Part model, mm, in its own coordinate system. Face numbers are marked on the shaded views. Round coordinates to 2 decimals unless told otherwise and drop trailing zeros. Loops run counter-clockwise (first coordinate to the right, second up) from the corner with the lowest first, then second, coordinate; pieces in that order, holes last. Notation, with made-up numbers: (11.25, 24.5) -> (60.25, 24.5) arc R27 ccw to (60.25, 63.5) -> close; hole circle Ø4 at (-32.75, 25.25). An arc over 180 degrees is marked (long way). Use a Markdown table: item, result. Add a question column.
Item 1: Probe line 1 (Z direction, x = 345, y = 43); line 2 (Y direction, x = 1050, z = -488.25); line 3 (Y direction, x = 960, z = -260). List the from-to ranges inside material, lowest first. Write a range as [from, to].
Item 2: Two-plate mould, pull along Z, no slides. Class the marked faces 1 and 2: pulls with the +Z half, pulls with the -Z half, needs draft (parallel to the pull), parting line crosses it, or undercut.
Item 3: Cut at A-A, the plane y = 30. List the corners of the cut face in (x, z).
Item 4: Cut at C-C, the plane x = 387.5. List the corners of the cut face in (y, z).
Item 5: Cut at B-B, the plane x = 1050. List the corners of the cut face in (y, z), plus the area to 3 significant figures.
Item 6: Flat gauge pin, fed straight in: pin 1 (1.5 mm diameter, centred on x = 274, z = -302.5, fed in from -Y). Where does the tip first touch, or does it go through?
Item 7: Cut at D-D, the plane z = -382. List the corners of the cut face in (x, y), plus the area to 3 significant figures.
```python
from build123d import *

# Parameters (mm, degrees)
SKETCH1_W           = 1200
SKETCH1_H           = 500
BOSS_EXTRUDE1_DEPTH = 68
SKETCH3_R           = 15
CUT_EXTRUDE2_DEPTH  = 1302.77724669
SKETCH4_R           = 15
CUT_EXTRUDE3_DEPTH  = 1302.77724669
SKETCH2_W           = 1200
SKETCH2_H           = 450
CUT_EXTRUDE1_DEPTH  = 50


with BuildPart() as part:
    # Sketch1 → Boss-Extrude1 (new body)
    with BuildSketch(Plane(origin=(0, 0, 0), x_dir=(1, 0, 0), z_dir=(0, 1, 0))):
        with Locations((600, 250)):
            Rectangle(SKETCH1_W, SKETCH1_H)
    extrude(amount=BOSS_EXTRUDE1_DEPTH)

    # Sketch3 → Cut-Extrude2 (cut, through all)
    with BuildSketch(Plane.XY):
        with Locations((150, 30)):
            Circle(SKETCH3_R)
    extrude(amount=-CUT_EXTRUDE2_DEPTH, mode=Mode.SUBTRACT)

    # Sketch4 → Cut-Extrude3 (cut, through all)
    with BuildSketch(Plane(origin=(0, 0, -500), x_dir=(-1, 0, 0), z_dir=(0, 0, -1))):
        with Locations((-1050, 30)):
            Circle(SKETCH4_R)
    extrude(amount=-CUT_EXTRUDE3_DEPTH, mode=Mode.SUBTRACT)

    # Sketch2 → Cut-Extrude1 (cut)
    with BuildSketch(Plane.XZ):
        with Locations((600, -250)):
            Rectangle(SKETCH2_W, SKETCH2_H)
    extrude(amount=-CUT_EXTRUDE1_DEPTH, mode=Mode.SUBTRACT)


solid = part.part
```
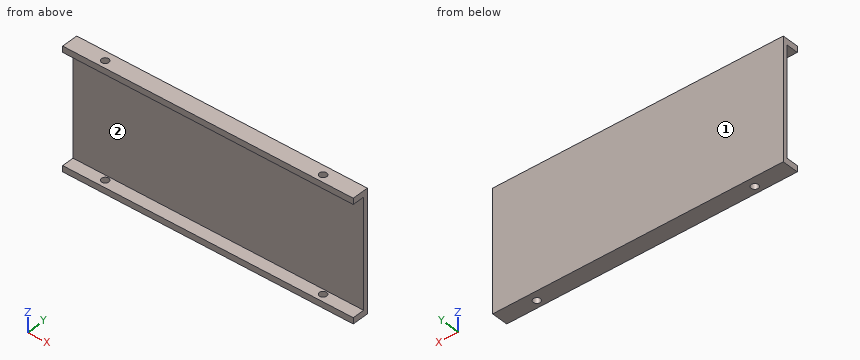
A:
| question | item | result |
|---|---|---|
| 1 | line 1 | z = [-500, -475], [-25, 0] |
| 1 | line 2 | y = [0, 15], [45, 68] |
| 1 | line 3 | y = [50, 68] |
| 2 | face 1 | needs draft |
| 2 | face 2 | undercut |
| 3 | outline | (0, -500) -> (135, -500) -> (135, -475) -> (0, -475) -> close; (0, -25) -> (135, -25) -> (135, 0) -> (0, 0) -> close; (165, -500) -> (1035, -500) -> (1035, -475) -> (165, -475) -> close; (165, -25) -> (1035, -25) -> (1035, 0) -> (165, 0) -> close; (1065, -500) -> (1200, -500) -> (1200, -475) -> (1065, -475) -> close; (1065, -25) -> (1200, -25) -> (1200, 0) -> (1065, 0) -> close |
| 4 | outline | (0, -500) -> (68, -500) -> (68, 0) -> (0, 0) -> (0, -25) -> (50, -25) -> (50, -475) -> (0, -475) -> close |
| 5 | outline | (0, -500) -> (15, -500) -> (15, -475) -> (0, -475) -> close; (0, -25) -> (15, -25) -> (15, 0) -> (0, 0) -> close; (45, -500) -> (68, -500) -> (68, 0) -> (45, 0) -> (45, -25) -> (50, -25) -> (50, -475) -> (45, -475) -> close |
| 5 | area | 10,000 mm^2 |
| 6 | pin 1 | stops at y = 50 |
| 7 | outline | (0, 50) -> (1200, 50) -> (1200, 68) -> (0, 68) -> close |
| 7 | area | 21,600 mm^2 |
